Input: part model. Units: mm. Frame: model coordinates. A direction names the side the tool comes from. Coordinates: 2 decimals unless noted, no trailing zeros. Use one line per item in the form item = value. Start each with the question number.
1) Access query for faces 1 (the flat face through (1, 14.3, -31.2)), 2 (the cylindrical face through (0, -0.2, -32.1)). Directions: +Z, -Z, +X, -X, +Y, -Y. A direction counts if a zero-diameter tool reaches every point of the face in a straight line with its end or side. Return the directions, or none.
2) Ray query, line 1 along Y through (x, z) = (-1.6, 0); line 2 along Z through (x, y) = (2.75, -20.5); line 3 along Z through (x, y) = (2.25, -7). Return the intervals inside material, ascending.
3) Pin query (flat end, axial travel): pin 1 (1.8 mm diameter, centred on x = 1, y = 23.5, fed in from +Z); pin 2 (3 mm diameter, centred on x = 0, y = -23, fed in from -Z). Return the tip coordinate at first contact, or that it passes through.
4) Section query B-B on y = 0. Count the separate pieces of the cut face and the enclosed holes in it, then the cut area to 3 significant figures.
from build123d import *

# Parameters (mm, degrees)
CUT_EXTRUDE2_DEPTH      = 58.026485075
FILLET1_R               = 0.5
CUT_EXTRUDE5_DEPTH      = 58.026485145
CUT_EXTRUDE5_DEPTH_BACK = 58.026485145
SKETCH7_R               = 4
SKETCH9_R               = 50
SKETCH9_R_2             = 34.1
CUT_EXTRUDE6_DEPTH      = 4


with BuildPart() as part:
    # Sketch1 → Revolve2 (revolve)
    with BuildSketch(Plane.XY, mode=Mode.PRIVATE) as revolve2_sk:
        Polygon((-3, 0), (-3, 38.05), (2, 38.05), (2, 40.1), (3, 40.1), (3, 0), align=None)
    revolve(revolve2_sk.sketch.rotate(Axis((3, 0, 0), (-1, 0, 0)), 90), axis=Axis((3, 0, 0), (-1, 0, 0)))

    # Sketch2 → Cut-Extrude2 (cut, through all)
    with BuildSketch(Plane.ZY.offset(-3)):
        with BuildLine():
            Line((14.415571014, 6.656167139), (27.571826318, 14.25193468))
            ThreePointArc((27.571826318, 14.25193468), (28.368418684, 14.340913448), (28.97445739, 13.816324366))
            ThreePointArc((28.97445739, 13.816324366), (32.1, 0), (28.97445739, -13.816324366))
            ThreePointArc((28.97445739, -13.816324366), (28.368418684, -14.340913448), (27.571826318, -14.25193468))
            Line((27.571826318, -14.25193468), (14.415571014, -6.656167139))
            ThreePointArc((14.415571014, -6.656167139), (13.972302174, -6.122171697), (13.983347826, -5.428257877))
            ThreePointArc((13.983347826, -5.428257877), (15, 0), (13.983347826, 5.428257877))
            ThreePointArc((13.983347826, 5.428257877), (13.972302174, 6.122171697), (14.415571014, 6.656167139))
        make_face()
        with BuildLine():
            Line((12.972195341, -9.156167139), (26.128450645, -16.75193468))
            ThreePointArc((26.128450645, -16.75193468), (26.603804702, -17.397314521), (26.452516582, -18.184453977))
            ThreePointArc((26.452516582, -18.184453977), (16.05, -27.799415461), (2.521940807, -32.000778343))
            ThreePointArc((2.521940807, -32.000778343), (1.764613982, -31.73822797), (1.443375673, -31.00386936))
            Line((1.443375673, -31.00386936), (1.443375673, -15.812334278))
            ThreePointArc((1.443375673, -15.812334278), (1.684194871, -15.161454481), (2.290664693, -14.824063386))
            ThreePointArc((2.290664693, -14.824063386), (7.5, -12.990381057), (11.692683133, -9.395805509))
            ThreePointArc((11.692683133, -9.395805509), (12.288107303, -9.039282784), (12.972195341, -9.156167139))
        make_face()
        with BuildLine():
            Line((-1.443375673, -15.812334278), (-1.443375673, -31.00386936))
            ThreePointArc((-1.443375673, -31.00386936), (-1.764613982, -31.73822797), (-2.521940807, -32.000778343))
            ThreePointArc((-2.521940807, -32.000778343), (-16.05, -27.799415461), (-26.452516582, -18.184453977))
            ThreePointArc((-26.452516582, -18.184453977), (-26.603804702, -17.397314521), (-26.128450645, -16.75193468))
            Line((-26.128450645, -16.75193468), (-12.972195341, -9.156167139))
            ThreePointArc((-12.972195341, -9.156167139), (-12.288107303, -9.039282784), (-11.692683133, -9.395805509))
            ThreePointArc((-11.692683133, -9.395805509), (-7.5, -12.990381057), (-2.290664693, -14.824063386))
            ThreePointArc((-2.290664693, -14.824063386), (-1.684194871, -15.161454481), (-1.443375673, -15.812334278))
        make_face()
        with BuildLine():
            Line((-14.415571014, -6.656167139), (-27.571826318, -14.25193468))
            ThreePointArc((-27.571826318, -14.25193468), (-28.368418684, -14.340913448), (-28.97445739, -13.816324366))
            ThreePointArc((-28.97445739, -13.816324366), (-32.1, 0), (-28.97445739, 13.816324366))
            ThreePointArc((-28.97445739, 13.816324366), (-28.368418684, 14.340913448), (-27.571826318, 14.25193468))
            Line((-27.571826318, 14.25193468), (-14.415571014, 6.656167139))
            ThreePointArc((-14.415571014, 6.656167139), (-13.972302174, 6.122171697), (-13.983347826, 5.428257877))
            ThreePointArc((-13.983347826, 5.428257877), (-15, 0), (-13.983347826, -5.428257877))
            ThreePointArc((-13.983347826, -5.428257877), (-13.972302174, -6.122171697), (-14.415571014, -6.656167139))
        make_face()
        with BuildLine():
            Line((-12.972195341, 9.156167139), (-26.128450645, 16.75193468))
            ThreePointArc((-26.128450645, 16.75193468), (-26.603804702, 17.397314521), (-26.452516582, 18.184453977))
            ThreePointArc((-26.452516582, 18.184453977), (-16.05, 27.799415461), (-2.521940807, 32.000778343))
            ThreePointArc((-2.521940807, 32.000778343), (-1.764613982, 31.73822797), (-1.443375673, 31.00386936))
            Line((-1.443375673, 31.00386936), (-1.443375673, 15.812334278))
            ThreePointArc((-1.443375673, 15.812334278), (-1.684194871, 15.161454481), (-2.290664693, 14.824063386))
            ThreePointArc((-2.290664693, 14.824063386), (-7.5, 12.990381057), (-11.692683133, 9.395805509))
            ThreePointArc((-11.692683133, 9.395805509), (-12.288107303, 9.039282784), (-12.972195341, 9.156167139))
        make_face()
        with BuildLine():
            Line((1.443375673, 15.812334278), (1.443375673, 31.00386936))
            ThreePointArc((1.443375673, 31.00386936), (1.764613982, 31.73822797), (2.521940807, 32.000778343))
            ThreePointArc((2.521940807, 32.000778343), (16.05, 27.799415461), (26.452516582, 18.184453977))
            ThreePointArc((26.452516582, 18.184453977), (26.603804702, 17.397314521), (26.128450645, 16.75193468))
            Line((26.128450645, 16.75193468), (12.972195341, 9.156167139))
            ThreePointArc((12.972195341, 9.156167139), (12.288107303, 9.039282784), (11.692683133, 9.395805509))
            ThreePointArc((11.692683133, 9.395805509), (7.5, 12.990381057), (2.290664693, 14.824063386))
            ThreePointArc((2.290664693, 14.824063386), (1.684194871, 15.161454481), (1.443375673, 15.812334278))
        make_face()
    extrude(amount=CUT_EXTRUDE2_DEPTH, mode=Mode.SUBTRACT)

    # Fillet1
    fillet1_edges = [part.edges().sort_by_distance(p)[0] for p in [
        (3, 0, 40.1),
        (2, 0, 40.1),
    ]]
    fillet(fillet1_edges, radius=FILLET1_R - 0.0001)  # a hair under: the kernel refuses the full size

    # Sketch7 → Cut-Extrude5 (cut, two sides: drawn at the far end of the back side and taken through both)
    with BuildSketch(Plane(origin=(3, 0, 0), x_dir=(0, 0, -1), z_dir=(1, 0, 0)).offset(-CUT_EXTRUDE5_DEPTH_BACK)):
        Circle(SKETCH7_R)
    extrude(amount=CUT_EXTRUDE5_DEPTH + CUT_EXTRUDE5_DEPTH_BACK, mode=Mode.SUBTRACT)

    # Sketch9 → Cut-Extrude6 (cut)
    with BuildSketch(Plane.ZY.offset(3)):
        Circle(SKETCH9_R)
        Circle(SKETCH9_R_2, mode=Mode.SUBTRACT)
    extrude(amount=-CUT_EXTRUDE6_DEPTH, mode=Mode.SUBTRACT)


solid = part.part
Answers below:
q1.face_1 = -X
q1.face_2 = +X, -X
q2.line_1 = -34.1 to -4, 4 to 34.1
q2.line_2 = -34.39 to -24.7, -1.44 to 1.44, 24.7 to 34.39
q2.line_3 = -39.42 to -31.33, -15.01 to 15.01, 31.33 to 39.42
q3.pin_1 = 30.61
q3.pin_2 = -31.13
q4.separate_pieces = 4
q4.enclosed_holes = 0
q4.area = 176 mm^2
